Design review of the part shown in the three views and the two pictorial views. Dimensions are in mm from the part's minimum x, y and z. A direction names the side the tool comes from. Give positions to 0.01 mm unless a question says otherwise; leave off trailing zeros. Write each loop counter-clockwise with the first axis right and the second up, starting at its lowest first coordinate (ties: lowest second). Pieces come first, ordered by that corner, then holes. Notation, with made-up numbers: (-15, -4.5) -> (35, -4.5) arc R28 cw to (35, 17.5) -> close; hole circle Ø7 at (52.25, 40). An arc over 180 degrees is marked (long way). Return JSON: item names as keys, results as strings. Group by question number.
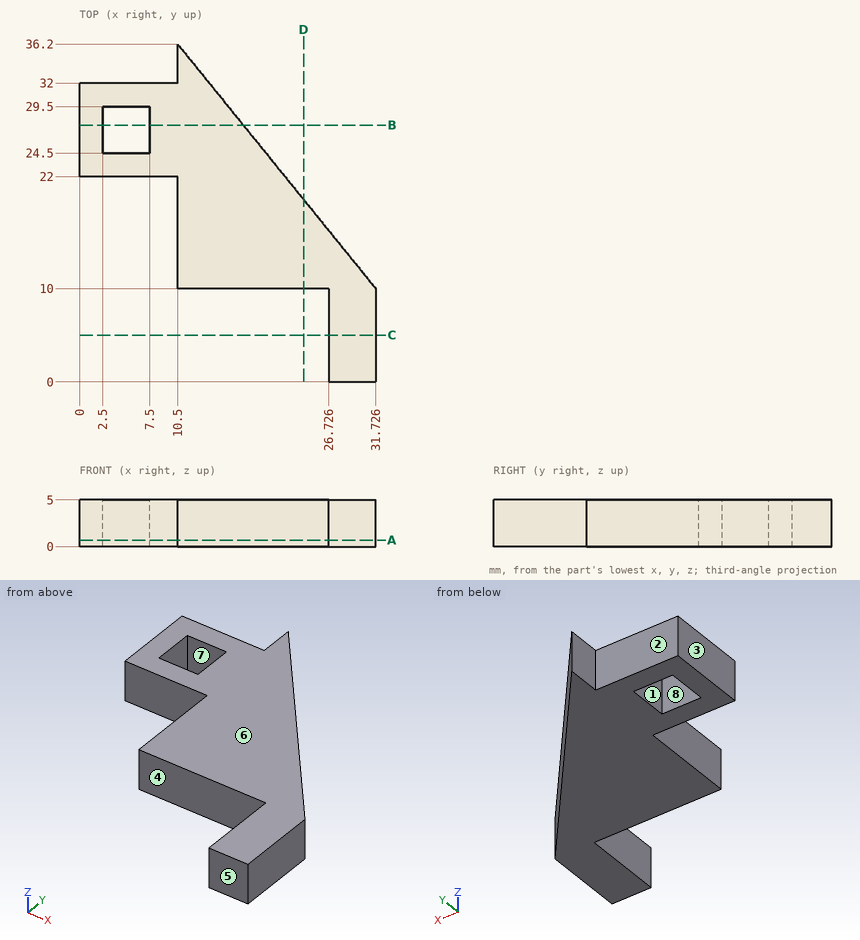
Q1. Take a section at C-C, the plane y = 5. Give the boundary of the cut face in (x, z).
Q2. Tool access review of the marked faces 1, 2, 3 and 4: name each direction out of +Z, -Z, +X, -X, +Y, -Y from which nothing blocks a thin tool from reaching the whole face with its end or side.
Q3. Mouldability with a two-part tool opening along Y and no side actions: class the marked faces 5, 6, 7 and 8 as +Y half, -Y half, draft (parallel to the pull), parting line (faces both ways), or undercut.
Q4. Insertion check: pin 1 (2 mm diameter, centred on x = 10, z = 1, fed in from +Y); pin 2 (1.5 mm diameter, centred on y = 7, z = 3, fed in from -X); pin 3 (1.5 mm diameter, centred on y = 27, z = 2, fed in from +X); pin 4 (2 mm diameter, centred on x = 28, y = 14.5, fed in from -Z). Each pin has a flat end and moves straight along its axis. Give the tip position at first contact, or say it passes through.
Q5. Take a section at A-A, the plane z = 0.7. Give the boundary of the cut face in (x, y).
Q6. Take a section at B-B, the plane y = 27.5. Give the boundary of the cut face in (x, z).
Q7. Take a section at D-D, the plane x = 24. Give the boundary of the cut face in (y, z), plus the area to 3 significant figures.
Q8. For L1, parallel to Y at x = 7, z = 2.05; L2, parallel to X at y = 6, z = 0.3; L3, parallel to Y at x = 22, z = 0.4 (1 decimal), list the stretches that pass through material, from the lowest coordinate up. Write a range as from..to.
Final values:
{
 "1": {"outline": "(26.73, 0) -> (31.73, 0) -> (31.73, 5) -> (26.73, 5) -> close"},
 "2": {"face 1": "+Z, -Z", "face 2": "+Z, -Z, -X, +Y", "face 3": "+Z, -Z, -X, +Y, -Y", "face 4": "+Z, -Z, -X, -Y"},
 "3": {"face 5": "-Y half", "face 6": "draft", "face 7": "undercut", "face 8": "undercut"},
 "4": {"pin 1": "stops at y = 36.2", "pin 2": "stops at x = 26.73", "pin 3": "stops at x = 18.56", "pin 4": "stops at z = 0"},
 "5": {"outline": "(0, 22) -> (10.5, 22) -> (10.5, 10) -> (26.73, 10) -> (26.73, 0) -> (31.73, 0) -> (31.73, 10) -> (10.5, 36.2) -> (10.5, 32) -> (0, 32) -> close; hole (2.5, 24.5) -> (7.5, 24.5) -> (7.5, 29.5) -> (2.5, 29.5) -> close"},
 "6": {"outline": "(0, 0) -> (2.5, 0) -> (2.5, 5) -> (0, 5) -> close; (7.5, 0) -> (17.55, 0) -> (17.55, 5) -> (7.5, 5) -> close"},
 "7": {"outline": "(10, 0) -> (19.54, 0) -> (19.54, 5) -> (10, 5) -> close", "area": "47.7 mm²"},
 "8": {"L1": "y = 22..24.5, 29.5..32", "L2": "x = 26.73..31.73", "L3": "y = 10..22"}
}
